from build123d import *

# Parameters (mm, degrees)
SKETCH_1_R               = 8.2
EXTRUDE_1_DEPTH          = 1
EXTRUDE_2_DEPTH          = 27
SKETCH_3_R               = 15
EXTRUDE_4_DEPTH          = 43
SKETCH_4_R               = 10
EXTRUDE_5_DEPTH          = 10
EXTRUDE_6_DEPTH          = 12
CUT_EXTRUDE_1_DEPTH      = 31
PATTERN_CIRCULAR_1_COUNT = 36
SKETCH_7_R               = 3
EXTRUDE_7_DEPTH          = 10
CUT_EXTRUDE_START        = -5
CUT_EXTRUDE_2_DEPTH      = 5
SKETCH_10_R              = 1.5
CUT_EXTRUDE_3_DEPTH      = 15


with BuildPart() as part:
    # 草图1 → 凸台-拉伸1 (new body)
    with BuildSketch(Plane(origin=(0, 0, 0), x_dir=(1, 0, 0), z_dir=(0, 1, 0))):
        with Locations(Location((0, 0, 0), (0, 0, 270))):
            Circle(SKETCH_1_R)
    extrude(amount=EXTRUDE_1_DEPTH)

    # 草图2 → 凸台-拉伸2 (add)
    with BuildSketch(Plane(origin=(0, 1, 0), x_dir=(1, 0, 0), z_dir=(0, 1, 0))):
        with BuildLine():
            ThreePointArc((16.20945122, -2.492727655), (18.9, 0), (16.20945122, 2.492727655))
            ThreePointArc((16.20945122, 2.492727655), (11.596551211, 11.596551211), (2.492727655, 16.20945122))
            ThreePointArc((2.492727655, 16.20945122), (0, 18.9), (-2.492727655, 16.20945122))
            ThreePointArc((-2.492727655, 16.20945122), (-11.596551211, 11.596551211), (-16.20945122, 2.492727655))
            ThreePointArc((-16.20945122, 2.492727655), (-18.9, 0), (-16.20945122, -2.492727655))
            ThreePointArc((-16.20945122, -2.492727655), (-11.596551211, -11.596551211), (-2.492727655, -16.20945122))
            ThreePointArc((-2.492727655, -16.20945122), (0, -18.9), (2.492727655, -16.20945122))
            ThreePointArc((2.492727655, -16.20945122), (11.596551211, -11.596551211), (16.20945122, -2.492727655))
        make_face()
    extrude(amount=EXTRUDE_2_DEPTH)

    # 草图3 → 凸台-拉伸4 (add)
    with BuildSketch(Plane(origin=(0, 28, 0), x_dir=(1, 0, 0), z_dir=(0, 1, 0))):
        with Locations(Location((0, 0, 0), (0, 0, 270))):
            Circle(SKETCH_3_R)
    extrude(amount=EXTRUDE_4_DEPTH)

    # 草图4 → 凸台-拉伸5 (add)
    with BuildSketch(Plane(origin=(0, 71, 0), x_dir=(1, 0, 0), z_dir=(0, 1, 0))):
        with Locations(Location((0, 0, 0), (0, 0, 270))):
            Circle(SKETCH_4_R)
    extrude(amount=EXTRUDE_5_DEPTH)

    # 草图5 → 凸台-拉伸6 (add)
    with BuildSketch(Plane(origin=(0, 71, 0), x_dir=(1, 0, 0), z_dir=(0, 1, 0))):
        with BuildLine():
            Line((-16.827061466, -4.806246186), (-4.806246186, -16.827061466))
            ThreePointArc((-4.806246186, -16.827061466), (12.374368671, -12.374368671), (16.827061466, 4.806246186))
            Line((16.827061466, 4.806246186), (4.806246186, 16.827061466))
            ThreePointArc((4.806246186, 16.827061466), (0, 17.5), (-4.806246186, 16.827061466))
            ThreePointArc((-4.806246186, 16.827061466), (-15.297058541, 8.5), (-16.827061466, -4.806246186))
        make_face()
    extrude(amount=-EXTRUDE_6_DEPTH)

    # 草图6 → 切除-拉伸1 (cut)
    with BuildSketch(Plane(origin=(0, 28, 0), x_dir=(1, 0, 0), z_dir=(0, 1, 0))):
        with BuildLine():
            ThreePointArc((-14.981238267, 0.75), (-15, 0), (-14.981238267, -0.75))
            Line((-14.981238267, -0.75), (-13.5, -0.75))
            Line((-13.5, -0.75), (-13.5, 0.75))
            Line((-13.5, 0.75), (-14.981238267, 0.75))
        make_face()
    cut_extrude_1 = extrude(amount=CUT_EXTRUDE_1_DEPTH, mode=Mode.SUBTRACT)

    # 阵列(圆周)1: 切除-拉伸1 ×36 about axis
    pattern_circular_1_axis = Axis((0, 0, 0), (0, 1, 0))
    for i in range(1, PATTERN_CIRCULAR_1_COUNT):
        add(cut_extrude_1.rotate(pattern_circular_1_axis, i * 360 / PATTERN_CIRCULAR_1_COUNT), mode=Mode.SUBTRACT)

    # 草图7 → 凸台-拉伸7 (add)
    with BuildSketch(Plane.XZ):
        with Locations(Location((0, 0, 0), (0, 0, 270))):
            Circle(SKETCH_7_R)
    extrude(amount=EXTRUDE_7_DEPTH)

    # 草图9 → 切除-拉伸2 (cut)
    with BuildSketch(Plane(origin=(0, -9, 0), x_dir=(-1, 0, 0), z_dir=(0, -1, 0)).offset(CUT_EXTRUDE_START)):
        with BuildLine():
            ThreePointArc((-3, 0), (-2.121320344, -2.121320344), (0, -3))
            Line((0, -3), (-3, 0))
        make_face()
        with BuildLine():
            ThreePointArc((0, -3), (2.121320344, -2.121320344), (3, 0))
            Line((3, 0), (0, -3))
        make_face()
    extrude(amount=CUT_EXTRUDE_2_DEPTH, mode=Mode.SUBTRACT)

    # 草图10 → 切除-拉伸3 (cut)
    with BuildSketch(Plane.XZ.offset(-1)):
        with Locations(Location((-8.485281374, -8.485281374, 0), (0, 0, 270))):
            Circle(SKETCH_10_R)
        with Locations(Location((-3.105828541, 11.591109915, 0), (0, 0, 270))):
            Circle(SKETCH_10_R)
        with Locations(Location((11.591109915, -3.105828541, 0), (0, 0, 270))):
            Circle(SKETCH_10_R)
    extrude(amount=-CUT_EXTRUDE_3_DEPTH, mode=Mode.SUBTRACT)


solid = part.part
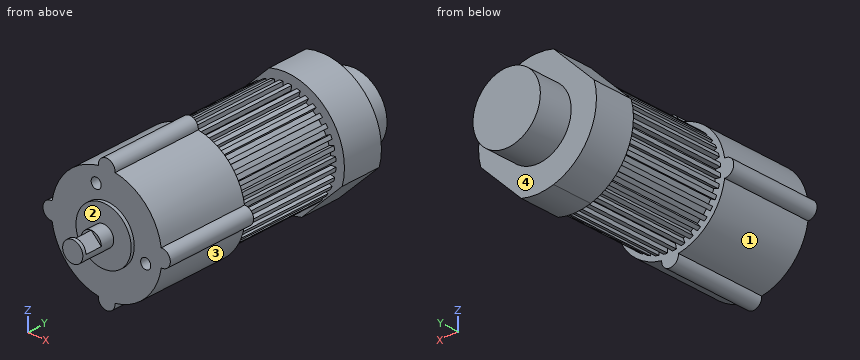
Can you work these out from the model? Positions are in its coordinate system, mm. Face numbers are marked on the shaded views. A direction names the side the tool comes from. Coordinates: 2 decimals unless noted, no trailing zeros. Loops run counter-clockwise (first coordinate to the right, second up) from the corner with the lowest first, then second, coordinate; pieces in that order, holes last. Notation, with made-up numbers: (-6.75, 74.5) - (44.25, 74.5) arc R20 ccw to (44.25, 88.5) - close; hole circle Ø5 at (-17, 85.5). An arc over 180 degrees is marked (long way). Put each result on its own line as item: value. Start each with the question number.
Item 1: If I drill on line 1 along Y through (x, z) = (2, 16.5); line 2 along Y through (x, z) = (17, -3); line 3 along Y through (x, z) = (-11, 7), over which ranges is the centre line in solid material (lowest first)?
Item 2: Which directions (+Z, -Z, +X, -X, +Y, -Y) give clear straight access to the entire face, cutting with the end or side of a thin tool? Please do the marked faces 1, 2, 3 and 4.
Item 3: Suppose I cut it at A-A (y = 24). Please give me the cut outline in (x, z).
Item 4: For pin 1 (5 mm diameter, centred on x = 8.5, z = -11, fed in from -Y); pin 2 (1.6 mm diameter, centred on x = 14.5, y = 50, fed in from -Z); pin 3 (1.6 mm diameter, centred on x = 0, y = 51, fed in from -Z), each with a flat end and sliding along its axis, tell me the tip position at first contact or that it passes through.
Item 5: Suppose I cut it at B-B (y = 64.5). Please give me the cut outline in (x, z).
Here are the results:
1. line 1: 1 to 28, 59 to 71
1. line 2: 59 to 71
1. line 3: 1 to 71
2. face 1: -Z, -X, -Y
2. face 2: -Y
2. face 3: -Z, +X, -Y
2. face 4: +Y
3. outline: (-16.21, -2.49) arc R16.4 ccw to (-2.49, -16.21) arc R2.5 ccw (long way) to (2.49, -16.21) arc R16.4 ccw to (16.21, -2.49) arc R2.5 ccw (long way) to (16.21, 2.49) arc R16.4 ccw to (2.49, 16.21) arc R2.5 ccw (long way) to (-2.49, 16.21) arc R16.4 ccw to (-16.21, 2.49) arc R2.5 ccw (long way) to start
4. pin 1: y = 1
4. pin 2: z = -6.11
4. pin 3: z = -14.98
5. outline: (-16.83, 4.81) arc R17.5 ccw to (4.81, -16.83) - (16.83, -4.81) arc R17.5 ccw to (-4.81, 16.83) - close
